from build123d import *

# Parameters (mm, degrees)
EXTRUDE_1_DEPTH = 15
SKETCH_2_R      = 6
EXTRUDE_2_DEPTH = 180


with BuildPart() as part:
    # 草图1 → 凸台-拉伸1 (new body)
    with BuildSketch(Plane(origin=(0, 0, 0), x_dir=(1, 0, 0), z_dir=(0, 1, 0))):
        Polygon((-7.216878365, 12.5), (-14.43375673, 0), (-7.216878365, -12.5), (7.216878365, -12.5), (14.43375673, 0), (7.216878365, 12.5), align=None)
    extrude(amount=-EXTRUDE_1_DEPTH)

    # 草图2 → 凸台-拉伸2 (add)
    with BuildSketch(Plane.XZ.offset(15)):
        with Locations(Location((0, 0, 0), (0, 0, 90))):
            Circle(SKETCH_2_R)
    extrude(amount=EXTRUDE_2_DEPTH)

    # 草图9 → 切除-旋转1 (revolve, cut)
    with BuildSketch(Plane.XY, mode=Mode.PRIVATE) as cut_revolve_1_sk:
        Polygon((11, 0), (14.43375673, -0.920072343), (14.43375673, 0), align=None)
    revolve(cut_revolve_1_sk.sketch.rotate(Axis((0, -195, 0), (0, 1, 0)), 90), axis=Axis((0, -195, 0), (0, 1, 0)), mode=Mode.SUBTRACT)


solid = part.part
Geometry: final body of the model. Coordinates: model frame, mm. A direction names the side the tool comes from. Give positions to 0.01 mm unless a question says otherwise; leave off trailing zeros. Loops run counter-clockwise (first coordinate to the right, second up) from the corner with the lowest first, then second, coordinate; pieces in that order, holes last. Notation, with made-up numbers: M 22,2 L 73,2 A23 cw 73,19 Z; hole C 9.25,-11 d5. An arc over 180 degrees is marked long. Put each result on its own line as item: value.
1) First-contact query: P1, Ø2, axis at x = -8, y = -76, coming from the +Z side; P2, Ø10, axis at x = 5, y = -120, coming from the +Z side; P3, Ø5, axis at x = 4.5, y = -63.5, coming from the -Z side; P4, Ø2, axis at x = -11.5, z = 5, coming from the -Y side. Flat tips, straight axial feed; report the tip coordinate or a pass-through.
Computed values:
P1: passes through
P2: stops at z = 6
P3: stops at z = -5.66
P4: stops at y = -15
2) Cut plane A-A, the plane x = 0. Return the cut outline in (y, z).
Computed values:
outline: M -195,-6 L -15,-6 L -15,-12.5 L -0.4,-12.5 L 0,-11 L 0,11 L -0.4,12.5 L -15,12.5 L -15,6 L -195,6 Z
3) Material intervals for L1, parallel to Y at x = 9.5, z = -2; L2, parallel to Y at x = 9.75, z = -8; L3, parallel to X at y = -175, z = 0, sorted ascending. Write a range as from..to.
Computed values:
L1: y = -15..0
L2: y = -15..-0.43
L3: x = -6..6
4) Reachability of faces 1 (the flat face through (-10.876, -7.599, 6.163)), 2 (the cylindrical face through (-1.802, -103.74, 5.723)) from +Z, -Z, +X, -X, +Y, -Y: full face, straight path, thin tool, end or side. Return the list, or none.
Computed values:
face 1: +Z, -X, +Y, -Y
face 2: -Y
5) Cut plane B-B, the plane y = -114.5. Return the cut outline in (x, z), plus the area to 3 significant figures.
Computed values:
outline: C 0,0 d12
area: 113 mm^2
